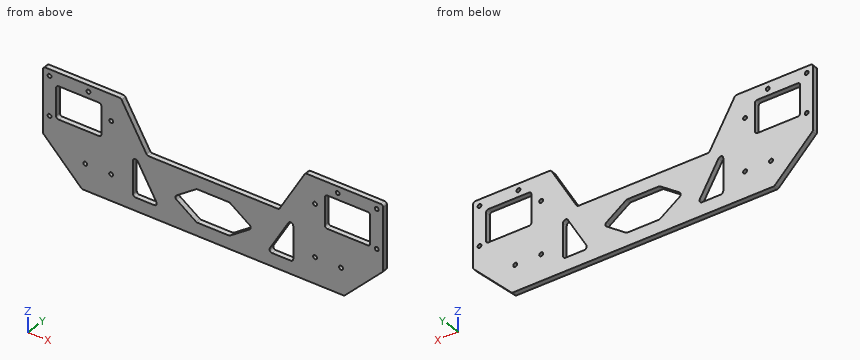
```python
from build123d import *

# Parameters (mm, degrees)
EXTRUDE_1_DEPTH     = 4
CUT_EXTRUDE_1_DEPTH = 4
CUT_EXTRUDE_2_DEPTH = 4
CUT_EXTRUDE_3_DEPTH = 4
FILLET_1_R          = 2
FILLET_2_R          = 2
SKETCH_5_R          = 1.5
CUT_EXTRUDE_4_DEPTH = 4
SKETCH_6_R          = 1.5
CUT_EXTRUDE_5_DEPTH = 4
SKETCH_7_R          = 1.5
CUT_EXTRUDE_6_DEPTH = 4
SKETCH_8_R          = 1.5
CUT_EXTRUDE_7_DEPTH = 4
SKETCH_9_R          = 1.5
CUT_EXTRUDE_8_DEPTH = 4
FILLET_3_R          = 2


with BuildPart() as part:
    # 草图1 → 凸台-拉伸1 (new body)
    with BuildSketch(Plane(origin=(0, 0, 0), x_dir=(1, 0, 0), z_dir=(0, 1, 0))):
        Polygon((65.54875717, -39.671128107), (125.54875717, -39.671128107), (125.54875717, 10.328871893), (95.54875717, 40.328871893), (-106.45124283, 40.328871893), (-136.45124283, 10.328871893), (-136.45124283, -39.671128107), (-76.45124283, -39.671128107), (-56.243983408, -4.671128107), (45.341497749, -4.671128107), align=None)
    extrude(amount=EXTRUDE_1_DEPTH)

    # 草图2 → 切除-拉伸1 (cut)
    with BuildSketch(Plane(origin=(0, 4, 0), x_dir=(1, 0, 0), z_dir=(0, 1, 0))):
        Polygon((7.216878365, 30.328871893), (-18.119364025, 30.328871893), (-35.90248566, 17.828871893), (-18.119364025, 5.328871893), (7.216878365, 5.328871893), (25, 17.828871893), align=None)
    extrude(amount=-CUT_EXTRUDE_1_DEPTH, mode=Mode.SUBTRACT)

    # 草图3 → 切除-拉伸2 (cut)
    with BuildSketch(Plane(origin=(0, 4, 0), x_dir=(1, 0, 0), z_dir=(0, 1, 0))):
        Polygon((-67.177653117, 30.328871893), (-47.429348489, 30.328871893), (-67.177653117, -3.876195086), align=None)
        Polygon((56.275167457, -3.876195086), (56.275167457, 30.328871893), (36.52686283, 30.328871893), align=None)
    extrude(amount=-CUT_EXTRUDE_2_DEPTH, mode=Mode.SUBTRACT)

    # 草图4 → 切除-拉伸3 (cut)
    with BuildSketch(Plane(origin=(0, 4, 0), x_dir=(1, 0, 0), z_dir=(0, 1, 0))):
        with BuildLine():
            Line((-124.45124283, -29.671128107), (-93.45124283, -29.671128107))
            ThreePointArc((-93.45124283, -29.671128107), (-92.037029267, -29.085341669), (-91.45124283, -27.671128107))
            Line((-91.45124283, -27.671128107), (-91.45124283, -6.671128107))
            ThreePointArc((-91.45124283, -6.671128107), (-92.037029267, -5.256914545), (-93.45124283, -4.671128107))
            Line((-93.45124283, -4.671128107), (-124.45124283, -4.671128107))
            ThreePointArc((-124.45124283, -4.671128107), (-125.865456392, -5.256914545), (-126.45124283, -6.671128107))
            Line((-126.45124283, -6.671128107), (-126.45124283, -27.671128107))
            ThreePointArc((-126.45124283, -27.671128107), (-125.865456392, -29.085341669), (-124.45124283, -29.671128107))
        make_face()
        with BuildLine():
            Line((115.54875717, -27.671128107), (115.54875717, -6.671128107))
            ThreePointArc((115.54875717, -6.671128107), (114.962970733, -5.256914545), (113.54875717, -4.671128107))
            Line((113.54875717, -4.671128107), (82.54875717, -4.671128107))
            ThreePointArc((82.54875717, -4.671128107), (81.134543608, -5.256914545), (80.54875717, -6.671128107))
            Line((80.54875717, -6.671128107), (80.54875717, -27.671128107))
            ThreePointArc((80.54875717, -27.671128107), (81.134543608, -29.085341669), (82.54875717, -29.671128107))
            Line((82.54875717, -29.671128107), (113.54875717, -29.671128107))
            ThreePointArc((113.54875717, -29.671128107), (114.962970733, -29.085341669), (115.54875717, -27.671128107))
        make_face()
    extrude(amount=-CUT_EXTRUDE_3_DEPTH, mode=Mode.SUBTRACT)

    # 圆角1
    fillet_1_edges = [part.edges().sort_by_distance(p)[0] for p in [
        (-67.177653117, 2, 3.876195086),
        (-67.177653117, 2, -30.328871893),
        (-47.429348489, 2, -30.328871893),
        (56.275167457, 2, 3.876195086),
        (36.52686283, 2, -30.328871893),
        (56.275167457, 2, -30.328871893),
    ]]
    fillet(fillet_1_edges, radius=FILLET_1_R)

    # 圆角2
    fillet_2_edges = [part.edges().sort_by_distance(p)[0] for p in [
        (-136.45124283, 2, -10.328871893),
        (-106.45124283, 2, -40.328871893),
        (95.54875717, 2, -40.328871893),
        (125.54875717, 2, -10.328871893),
        (125.54875717, 2, 39.671128107),
        (65.54875717, 2, 39.671128107),
        (45.341497749, 2, 4.671128107),
        (-56.243983408, 2, 4.671128107),
        (-76.45124283, 2, 39.671128107),
        (-136.45124283, 2, 39.671128107),
    ]]
    fillet(fillet_2_edges, radius=FILLET_2_R)

    # 草图5 → 切除-拉伸4 (cut)
    with BuildSketch(Plane(origin=(0, 4, 0), x_dir=(1, 0, 0), z_dir=(0, 1, 0))):
        with Locations(Location((73.04875717, -19.671128107, 0), (0, 0, 270))):
            Circle(SKETCH_5_R)
        with Locations(Location((73.04875717, 20.328871893, 0), (0, 0, 270))):
            Circle(SKETCH_5_R)
        with Locations(Location((-83.95124283, -19.671128107, 0), (0, 0, 90))):
            Circle(SKETCH_5_R)
        with Locations(Location((-83.95124283, 20.328871893, 0), (0, 0, 90))):
            Circle(SKETCH_5_R)
    extrude(amount=-CUT_EXTRUDE_4_DEPTH, mode=Mode.SUBTRACT)

    # 草图6 → 切除-拉伸5 (cut)
    with BuildSketch(Plane(origin=(0, 4, 0), x_dir=(1, 0, 0), z_dir=(0, 1, 0))):
        with Locations(Location((120.54875717, -34.671128107, 0), (0, 0, 270))):
            Circle(SKETCH_6_R)
        with Locations(Location((93.04875717, 20.328871893, 0), (0, 0, 270))):
            Circle(SKETCH_6_R)
        with Locations(Location((90.54875717, -34.671128107, 0), (0, 0, 270))):
            Circle(SKETCH_6_R)
    extrude(amount=-CUT_EXTRUDE_5_DEPTH, mode=Mode.SUBTRACT)

    # 草图7 → 切除-拉伸6 (cut)
    with BuildSketch(Plane(origin=(0, 4, 0), x_dir=(1, 0, 0), z_dir=(0, 1, 0))):
        with Locations(Location((120.54875717, -4.671128107, 0), (0, 0, 270))):
            Circle(SKETCH_7_R)
    extrude(amount=-CUT_EXTRUDE_6_DEPTH, mode=Mode.SUBTRACT)

    # 草图8 → 切除-拉伸7 (cut)
    with BuildSketch(Plane(origin=(0, 4, 0), x_dir=(1, 0, 0), z_dir=(0, 1, 0))):
        with Locations(Location((-131.45124283, -34.671128107, 0), (0, 0, 270))):
            Circle(SKETCH_8_R)
        with Locations(Location((-101.45124283, -34.671128107, 0), (0, 0, 270))):
            Circle(SKETCH_8_R)
        with Locations(Location((-131.45124283, -4.671128107, 0), (0, 0, 270))):
            Circle(SKETCH_8_R)
    extrude(amount=-CUT_EXTRUDE_7_DEPTH, mode=Mode.SUBTRACT)

    # 草图9 → 切除-拉伸8 (cut)
    with BuildSketch(Plane(origin=(0, 4, 0), x_dir=(1, 0, 0), z_dir=(0, 1, 0))):
        with Locations(Location((-103.95124283, 20.328871893, 0), (0, 0, 270))):
            Circle(SKETCH_9_R)
    extrude(amount=-CUT_EXTRUDE_8_DEPTH, mode=Mode.SUBTRACT)

    # 圆角3
    fillet_3_edges = [part.edges().sort_by_distance(p)[0] for p in [
        (7.216878365, 2, -30.328871893),
        (25, 2, -17.828871893),
        (7.216878365, 2, -5.328871893),
        (-18.119364025, 2, -5.328871893),
        (-35.90248566, 2, -17.828871893),
        (-18.119364025, 2, -30.328871893),
    ]]
    fillet(fillet_3_edges, radius=FILLET_3_R)


solid = part.part
```
Source: CAD feature listing. Evaluate the final solid. Frame: model axes, mm. Coordinates: 2 decimals unless noted, no trailing zeros. Write each loop counter-clockwise with the first axis right and the second up, starting at its lowest first coordinate (ties: lowest second). Pieces come first, ordered by that corner, then holes. Notation, with made-up numbers: M 72,70 L 118,70 A25 cw 118,98 Z; hole C -34,-8.75 d11. An arc over 180 degrees is marked long. Answer as a JSON object with one key per item and string values.
1. Cut plane B-B on y = 3.2. State how many separate pieces and enclosed holes the cut face has, plus the area to 3 significant figures.
Evaluation:
{"separate pieces": "1", "enclosed holes": "17", "area": "12,200 mm^2"}
2. Cut plane A-A on z = 11. Output: boundary loops of the cut face in (x, y).
Evaluation:
{"outline": "M -136.45,0 L -126.45,0 L -126.45,4 L -136.45,4 Z; M -91.45,0 L -59.9,0 L -59.9,4 L -91.45,4 Z; M 49,0 L 80.55,0 L 80.55,4 L 49,4 Z; M 115.55,0 L 125.55,0 L 125.55,4 L 115.55,4 Z"}
3. Contact query for flat-ended pins moving along their axis: P1, Ø1.2, axis at y = 1, z = -19.5, coming from the +X side; P2, Ø1.5, axis at x = 32.5, y = 3, coming from the +Z side. Output: stop coordinate, or through.
Evaluation:
{"P1": "x = 116.98", "P2": "z = 4.67"}
4. Ray query, L1, parallel to X at y = 3.8, z = -30; L2, parallel to X at y = 0.4, z = -24.5; L3, parallel to Z at x = 0, y = 0.35. Return the intervals inside material, ascending.
Evaluation:
{"L1": "-116.78 to -66.28, -49.79 to -18.59, 7.68 to 38.89, 55.37 to 105.88", "L2": "-122.28 to -67.18, -50.79 to -26.41, 15.51 to 39.89, 56.28 to 111.38", "L3": "-40.33 to -30.33, -5.33 to 4.67"}
